Check sheet for the modelled part. Datum: model origin and axes. Units: mm. Round coordinates to 2 decimals unless told otherwise and drop trailing zeros. Order: outer loops, then holes, each group sorted by start corner. A loop starts at its lowest first (then second) coordinate and runs counter-clockwise, first axis right, second up. Notation, with made-up numbers: M 12.25,16 L 52.25,16 A12 ccw 52.25,26 Z; hole C 71.25,39.5 d5. An arc over 180 degrees is marked long. One line per item, written item: value. Start each with the question number.
(1) Thickness scan on L1, parallel to Z at x = 0.3, y = -1; L2, parallel to Y at x = 0.3, z = 0.85; L3, parallel to Z at x = 0.05, y = 6.25. Record the ranges inside material, lowest first.
(2) Cross-section at D-D, the plane y = 5. Enter the section's corners in (x, z), and give its area (3 significant figures).
(3) Cross-section at C-C, the plane y = 0. Enter the section's corners in (x, z), and give its area (3 significant figures).
(4) Cross-section at B-B, the plane x = 0.1. Enter the section's corners in (y, z).
(5) Cross-section at A-A, the plane y = 6.25. Enter the section's corners in (x, z), and give its area (3 significant figures).
from build123d import *

# Parameters (mm, degrees)
BOSS_EXTRUDE1_DEPTH = 0.4


with BuildPart() as part:
    # Sketch1 → Boss-Extrude1 (new body)
    with BuildSketch(Plane(origin=(0, 0, 0), x_dir=(0, 0, -1), z_dir=(1, 0, 0))):
        with BuildLine():
            Line((-0.486576567, 7.906439428), (-0.277438328, 2.156274237))
            Line((-0.277438328, 2.156274237), (-0.518351631, 1.906439428))
            Line((-0.518351631, 1.906439428), (-1.019947879, 1.906439428))
            Line((-1.019947879, 1.906439428), (-1.019947879, -1.820037787))
            ThreePointArc((-1.019947879, -1.820037787), (-1.060356555, -1.956314993), (-1.168519693, -2.048537947))
            Line((-1.168519693, -2.048537947), (-1.269947879, -2.093560572))
            Line((-1.269947879, -2.093560572), (-1.371376066, -2.048537947))
            ThreePointArc((-1.371376066, -2.048537947), (-1.479539204, -1.956314993), (-1.519947879, -1.820037787))
            Line((-1.519947879, -1.820037787), (-1.519947879, 1.906439428))
            Line((-1.519947879, 1.906439428), (-2.021544128, 1.906439428))
            Line((-2.021544128, 1.906439428), (-2.26245743, 2.156274237))
            Line((-2.26245743, 2.156274237), (-2.053319191, 7.906439428))
            Line((-2.053319191, 7.906439428), (-1.594947879, 7.296916042))
            Line((-1.594947879, 7.296916042), (-1.785118415, 6.950118253))
            Line((-1.785118415, 6.950118253), (-1.785185155, 3.40759606))
            ThreePointArc((-1.785185155, 3.40759606), (-1.681017639, 3.102108908), (-1.411909463, 2.923912215))
            Line((-1.411909463, 2.923912215), (-1.269947879, 2.886717808))
            Line((-1.269947879, 2.886717808), (-1.127986296, 2.923912215))
            ThreePointArc((-1.127986296, 2.923912215), (-0.85887812, 3.102108908), (-0.754710604, 3.40759606))
            Line((-0.754710604, 3.40759606), (-0.754777344, 6.950118253))
            Line((-0.754777344, 6.950118253), (-0.944947879, 7.296916042))
            Line((-0.944947879, 7.296916042), (-0.486576567, 7.906439428))
        make_face()
    extrude(amount=BOSS_EXTRUDE1_DEPTH)


solid = part.part
Values found:
1. L1: 1.02 to 1.52
1. L2: 1.91 to 3.11, 7.12 to 7.42
1. L3: 0.43 to 0.75, 1.79 to 2.11
2. outline: M 0,0.38 L 0.4,0.38 L 0.4,0.75 L 0,0.75 Z; M 0,1.79 L 0.4,1.79 L 0.4,2.16 L 0,2.16 Z
2. area: 0.299 mm^2
3. outline: M 0,1.02 L 0.4,1.02 L 0.4,1.52 L 0,1.52 Z
3. area: 0.200 mm^2
4. outline: M -2.09,1.27 L -2.05,1.17 A0.25 ccw -1.82,1.02 L 1.91,1.02 L 1.91,0.52 L 2.16,0.28 L 7.91,0.49 L 7.3,0.94 L 6.95,0.75 L 3.41,0.75 A0.5 cw 2.92,1.13 L 2.89,1.27 L 2.92,1.41 A0.5 cw 3.41,1.79 L 6.95,1.79 L 7.3,1.59 L 7.91,2.05 L 2.16,2.26 L 1.91,2.02 L 1.91,1.52 L -1.82,1.52 A0.25 ccw -2.05,1.37 Z
5. outline: M 0,0.43 L 0.4,0.43 L 0.4,0.75 L 0,0.75 Z; M 0,1.79 L 0.4,1.79 L 0.4,2.11 L 0,2.11 Z
5. area: 0.263 mm^2
